CAD build for the part. Positions are in the model's coordinates, mm. Face numbers are marked on the shaded views. A direction names the side the tool comes from. Give positions to 0.01 mm unless a question says otherwise; leave off trailing zeros. Order: outer loops, then holes, each group sorted by start corner. A loop starts at its lowest first (then second) coordinate and runs counter-clockwise, first axis right, second up.
Item 1: Wall check: L1, parallel to X at y = -0.5, z = 1.4; L2, parallel to Z at x = -3.5, y = -1.75; L3, parallel to Y at x = -15.25, z = 1.2. Give the ranges that are in metal, low to high.
Item 2: Band-saw the part on D-D on z = 1.35. Give the cut face in (x, y).
Item 3: Band-saw the part on B-B on z = 2.6. Give the cut face in (x, y), plus the area to 3 significant figures.
Item 4: Two-plate mould, pull along Y, no slides. Class the marked faces 3, 4, 5 and 6: released by +Y, released by -Y, zero draft, split by the parting line, or undercut.
Item 5: Flat gauge pins, fed straight in: P1, Ø2.5, axis at x = -3.95, y = 0, coming from the +Z side; P2, Ø0.6, axis at y = -0.5, z = 2.5, coming from the +X side; P3, Ø3, axis at x = -15.94, y = 0, coming from the +Z side (3 decimals). Where does each tip first touch, or does it go through?
Item 6: Which spindle directions (+Z, -Z, +X, -X, +Y, -Y) get a long thin tool onto all of the face, cutting with end or side? Do the marked faces 1 and 2. Say none if no direction does.
Item 7: Band-saw the part on A-A on y = 0. Give the cut face in (x, z), plus the area to 3 significant figures.
Item 8: Band-saw the part on C-C on x = -14.5. Give the cut face in (y, z), plus the area to 3 significant figures.
```python
from build123d import *

# Parameters (mm, degrees)
IZIM1_R                     = 1.6
IZIM1_R_2                   = 1
Y_KSEKLIK_EKSTR_ZYON1_DEPTH = 3
IZIM2_W                     = 1.154616757
IZIM2_H                     = 7
KES_EKSTR_ZYON1_DEPTH       = 11.5


with BuildPart() as part:
    # Çizim1 → Yükseklik-Ekstrüzyon1 (new body)
    with BuildSketch(Plane.XY):
        with BuildLine():
            Line((-19.5, 0.5), (-19.5, -0.5))
            ThreePointArc((-19.5, -0.5), (-18.621320344, -2.621320344), (-16.5, -3.5))
            Line((-16.5, -3.5), (-5.048446869, -3.5))
            ThreePointArc((-5.048446869, -3.5), (-3.176019241, -2.843931479), (-2.122552163, -1.162676519))
            Line((-2.122552163, -1.162676519), (-2.009308765, -0.662676519))
            ThreePointArc((-2.009308765, -0.662676519), (-1.935203471, 0), (-2.009308765, 0.662676519))
            Line((-2.009308765, 0.662676519), (-2.122552163, 1.162676519))
            ThreePointArc((-2.122552163, 1.162676519), (-3.176019241, 2.843931479), (-5.048446869, 3.5))
            Line((-5.048446869, 3.5), (-16.5, 3.5))
            ThreePointArc((-16.5, 3.5), (-18.621320344, 2.621320344), (-19.5, 0.5))
        make_face()
        with Locations((-15.940902873, 0)):
            Circle(IZIM1_R, mode=Mode.SUBTRACT)
        with Locations((-3.94869662, 0)):
            Circle(IZIM1_R_2, mode=Mode.SUBTRACT)
    extrude(amount=Y_KSEKLIK_EKSTR_ZYON1_DEPTH)

    # Çizim2 → Kes-Ekstrüzyon1 (cut, symmetric)
    with BuildSketch(Plane(origin=(0, 0, 0), x_dir=(0, 0, -1), z_dir=(1, 0, 0))):
        with Locations((-2.422691622, 0)):
            Rectangle(IZIM2_W, IZIM2_H)
    extrude(amount=KES_EKSTR_ZYON1_DEPTH, both=True, mode=Mode.SUBTRACT)


solid = part.part
```
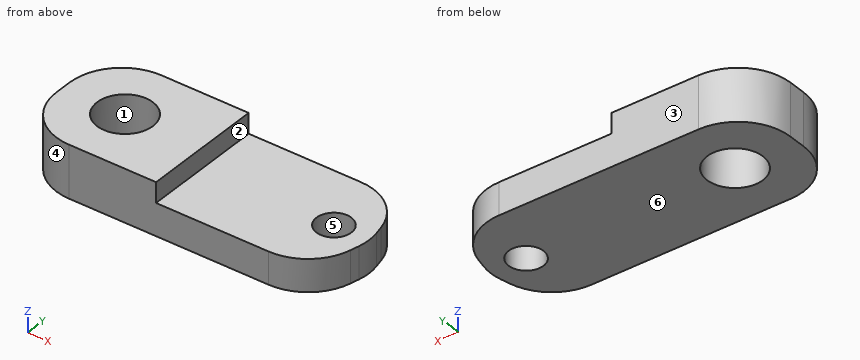
The answers:
1. L1: x = -19.5 to -17.46, -14.42 to -4.81, -3.08 to -1.98
1. L2: z = 0 to 1.85
1. L3: y = -3.5 to -1.44, 1.44 to 3.5
2. outline: (-19.5, -0.5) arc R3 ccw to (-16.5, -3.5) - (-5.05, -3.5) arc R3 ccw to (-2.12, -1.16) - (-2.01, -0.66) arc R3 ccw to (-2.01, 0.66) - (-2.12, 1.16) arc R3 ccw to (-5.05, 3.5) - (-16.5, 3.5) arc R3 ccw to (-19.5, 0.5) - close; hole circle Ø3.2 at (-15.94, 0); hole circle Ø2 at (-3.95, 0)
3. outline: (-19.5, -0.5) arc R3 ccw to (-16.5, -3.5) - (-11.5, -3.5) - (-11.5, 3.5) - (-16.5, 3.5) arc R3 ccw to (-19.5, 0.5) - close; hole circle Ø3.2 at (-15.94, 0)
3. area: 44.1 mm2
4. face 3: released by +Y
4. face 4: released by -Y
4. face 5: undercut
4. face 6: zero draft
5. P1: stops at z = 1.85
5. P2: stops at x = -11.5
5. P3: passes through
6. face 1: +Z, -Z
6. face 2: +Z, +X, +Y, -Y
7. outline: (-19.5, 0) - (-17.54, 0) - (-17.54, 3) - (-19.5, 3) - close; (-14.34, 0) - (-4.95, 0) - (-4.95, 1.85) - (-11.5, 1.85) - (-11.5, 3) - (-14.34, 3) - close; (-2.95, 0) - (-1.94, 0) - (-1.94, 1.85) - (-2.95, 1.85) - close
7. area: 28.4 mm2
8. outline: (-3.5, 0) - (-0.7, 0) - (-0.7, 3) - (-3.5, 3) - close; (0.7, 0) - (3.5, 0) - (3.5, 3) - (0.7, 3) - close
8. area: 16.8 mm2
